Can you work these out from the model? Positions are in its coordinate system, mm. Give positions to 0.01 mm unless a question says otherwise; leave off trailing zeros. Write each loop counter-clockwise with the first axis right and the second up, starting at its lowest first coordinate (ties: lowest second). Pieces come first, ordered by that corner, then holes.
1. I'm going to push flat-ended pins straight in: pin 1 (1.5 mm diameter, centred on x = 6.5, y = 15, fed in from +Z); pin 2 (6 mm diameter, centred on x = -2.5, y = 13, fed in from +Z); pin 3 (10 mm diameter, centred on y = 21.5, z = 23.5, fed in from -X) (3 decimals); pin 4 (12 mm diameter, centred on x = 5.5, y = 14, fed in from +Z). Where does each tip first touch, or does it pass through?
2. Suppose I cut it at A-A (z = 4). Please give me the cut outline in (x, y), and give its area (3 significant figures).
3. If I drill on probe 1 along Z at (x, y) = (-9, 5); probe 2 along X at (y, z) = (6.5, 27); probe 3 along Y at (x, z) = (-1, 32.5), over which ranges is the centre line in solid material (lowest first)?
```python
from build123d import *

# Parameters (mm, degrees)
F0_R     = 25.4
F1_DEPTH = 50.8
F2_SIZE2 = 50.79999
F2_SIZE  = 25.39999
F3_W     = 50.8
F3_H     = 25.4
F4_DEPTH = 101


# Not quite as in the source:
# - a fillet or chamfer is up to 0.001 mm smaller than in the source, because OpenCascade refuses the exact size
# - an extrude ends at something that could not be found from the text; its depth is read off the source's solid


with BuildPart() as f1:
    # F0 (on Top) → F1 (new body)
    with BuildSketch(Plane.XY):
        Circle(F0_R)
    extrude(amount=F1_DEPTH)

    # F2 (size 25.4 and 50.8 in the source; OpenCascade refuses exactly that, so slightly less here)
    f2_edges = [f1.edges().sort_by_distance(p)[0] for p in [
        (-25.4, 0, 50.8),
    ]]
    f2_side = f1.faces().sort_by_distance((0, 0, 50.8))[0]
    chamfer(f2_edges, length=F2_SIZE, length2=F2_SIZE2, reference=f2_side)

    # F3 (on face) → F4 (cut, through all)
    with BuildSketch(Plane(origin=(0, 0, 0), x_dir=(1, 0, 0), z_dir=(0, 0, -1))):
        with Locations((0, 12.7)):
            Rectangle(F3_W, F3_H)
    extrude(amount=-F4_DEPTH, mode=Mode.SUBTRACT)


solid = f1.part
```
Checks:
1. pin 1: stops at z = 19.6
1. pin 2: stops at z = 30.32
1. pin 3: passes through
1. pin 4: stops at z = 32.72
2. outline: (-23.4, 0) - (23.4, 0) arc R23.4 ccw to start
2. area: 860 mm2
3. probe 1: z = 0 to 30.21
3. probe 2: x = -9.97 to 9.97
3. probe 3: y = 0 to 9.1
